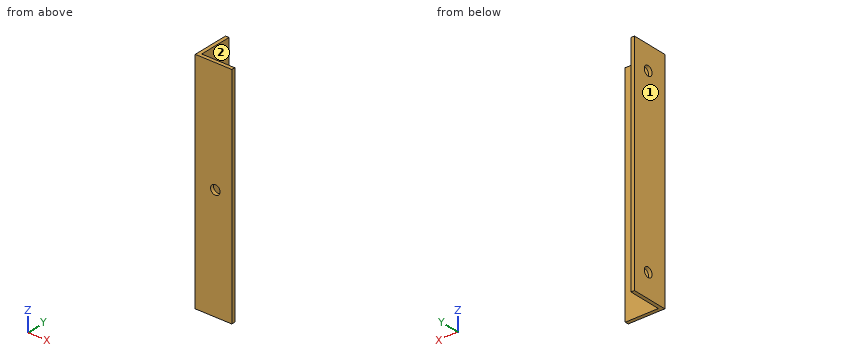
```python
from build123d import *

# Parameters (mm, degrees)
EXTRU_MINCE1_DEPTH      = 96
ESQUISSE2_R             = 2
ENL_V_MAT_EXTRU_1_DEPTH = 99.245865053
ESQUISSE3_R             = 2
ENL_V_MAT_EXTRU_2_DEPTH = 99.245865053


with BuildPart() as part:
    # Esquisse1 → Extru.-Mince1 (new body)
    with BuildSketch(Plane.XY):
        Polygon((0, 15.5), (0, 0), (15.5, 0), (15.5, 1.5), (1.5, 1.5), (1.5, 15.5), align=None)
    extrude(amount=EXTRU_MINCE1_DEPTH)

    # Esquisse2 → Enlèv. mat.-Extru.1 (cut, through all)
    with BuildSketch(Plane(origin=(1.5, 0, 0), x_dir=(0, 0, -1), z_dir=(1, 0, 0))):
        with Locations(Location((-86, 8.5, 0), (0, 0, 90))):
            Circle(ESQUISSE2_R)
        with Locations(Location((-10, 8.5, 0), (0, 0, 270))):
            Circle(ESQUISSE2_R)
    extrude(amount=-ENL_V_MAT_EXTRU_1_DEPTH, mode=Mode.SUBTRACT)

    # Esquisse3 → Enlèv. mat.-Extru.2 (cut, through all)
    with BuildSketch(Plane(origin=(0, 1.5, 0), x_dir=(1, 0, 0), z_dir=(0, 1, 0))):
        with Locations(Location((8.5, -48, 0), (0, 0, 270))):
            Circle(ESQUISSE3_R)
    extrude(amount=-ENL_V_MAT_EXTRU_2_DEPTH, mode=Mode.SUBTRACT)


solid = part.part
```
Model file for the job. Use its own axes, mm. Face numbers are marked on the shaded views. A direction names the side the tool comes from. Give positions to 0.01 mm unless a question says otherwise; leave off trailing zeros. Loops run counter-clockwise (first coordinate to the right, second up) from the corner with the lowest first, then second, coordinate; pieces in that order, holes last. Notation, with made-up numbers: (5.25, 46) -> (61.25, 46) arc R28 cw to (61.25, 69) -> close; hole circle Ø7 at (23.25, 79.25). An arc over 180 degrees is marked (long way). Write each question's results on one line, items separated by ' | '.
(1) Tool access for the marked faces 1 and 2: list every direction of +Z, -Z, +X, -X, +Y, -Y with a clear straight run to the whole face (end or side of a thin tool).
Geometry results:
face 1: +Z, -Z, -X, +Y, -Y | face 2: +Z, -Z, +X, +Y
(2) Cut at A-A on z = 86. List the corners of the cut face in (x, y).
Geometry results:
outline: (0, 0) -> (15.5, 0) -> (15.5, 1.5) -> (1.5, 1.5) -> (1.5, 6.5) -> (0, 6.5) -> close; (0, 10.5) -> (1.5, 10.5) -> (1.5, 15.5) -> (0, 15.5) -> close
(3) Cut at C-C on y = 8.5. List the corners of the cut face in (x, z), and give its area (3 significant figures).
Geometry results:
outline: (0, 0) -> (1.5, 0) -> (1.5, 8) -> (0, 8) -> close; (0, 12) -> (1.5, 12) -> (1.5, 84) -> (0, 84) -> close; (0, 88) -> (1.5, 88) -> (1.5, 96) -> (0, 96) -> close | area: 132 mm²
(4) Probe line 1 along Z through (x, y) = (0.5, 8.5); line 2 along Y through (x, z) = (0.4, 10). List the from-to ranges inside material, lowest first.
Geometry results:
line 1: z = 0 to 8, 12 to 84, 88 to 96 | line 2: y = 0 to 6.5, 10.5 to 15.5
(5) Cut at D-D on z = 63.5. List the corners of the cut face in (x, y), and give its area (4 significant figures).
Geometry results:
outline: (0, 0) -> (15.5, 0) -> (15.5, 1.5) -> (1.5, 1.5) -> (1.5, 15.5) -> (0, 15.5) -> close | area: 44.25 mm²
(6) Cut at B-B on x = 8.5. List the corners of the cut face in (y, z), and give its area (3 significant figures).
Geometry results:
outline: (0, 0) -> (1.5, 0) -> (1.5, 46) -> (0, 46) -> close; (0, 50) -> (1.5, 50) -> (1.5, 96) -> (0, 96) -> close | area: 138 mm²
(7) Flat gauge pins, fed straight in: pin 1 Ø4 at (y, z) = (2, 45.5) entering from +X; pin 2 Ø1.5 at (y, z) = (9.5, 13.5) entering from +X; pin 3 Ø4 at (x, z) = (5, 64.5) entering from +Y. Where does each tip first touch, or does it go through?
Geometry results:
pin 1: stops at x = 15.5 | pin 2: stops at x = 1.5 | pin 3: stops at y = 1.5
